from build123d import *

# Parameters (mm, degrees)
SKETCH_1_R      = 2.5
EXTRUDE_1_DEPTH = 4


with BuildPart() as part:
    # 草图1 → 凸台-拉伸1 (new body)
    with BuildSketch(Plane.XY):
        with BuildLine():
            Line((-3.705318961, 51.777526587), (-4.499753228, 50.342391759))
            ThreePointArc((-4.499753228, 50.342391759), (-4.72372629, 49.780297575), (-4.8, 49.180050853))
            Line((-4.8, 49.180050853), (-4.8, 14.202498322))
            ThreePointArc((-4.8, 14.202498322), (-4.74482021, 13.6908166), (-4.581818179, 13.20266362))
            Line((-4.581818179, 13.20266362), (-4.112355754, 12.178212626))
            ThreePointArc((-4.112355754, 12.178212626), (-3.746152658, 10.910853721), (-3.111838791, 9.754156171))
            ThreePointArc((-3.111838791, 9.754156171), (-2.4, 7.5), (-3.111838791, 5.245843829))
            ThreePointArc((-3.111838791, 5.245843829), (-3.921495991, 3.606788208), (-4.2, 1.8))
            Line((-4.2, 1.8), (-4.2, 0))
            ThreePointArc((-4.2, 0), (0, -4.2), (4.2, 0))
            Line((4.2, 0), (4.2, 1.8))
            ThreePointArc((4.2, 1.8), (3.921495991, 3.606788208), (3.111838791, 5.245843829))
            ThreePointArc((3.111838791, 5.245843829), (2.4, 7.5), (3.111838791, 9.754156171))
            ThreePointArc((3.111838791, 9.754156171), (3.921495991, 11.393211792), (4.2, 13.2))
            Line((4.2, 13.2), (4.2, 49.8))
            ThreePointArc((4.2, 49.8), (1.019230191, 53.874453315), (-3.705318961, 51.777526587))
        make_face()
        Circle(SKETCH_1_R, mode=Mode.SUBTRACT)
        with BuildLine():
            Line((-3, 45.643078062), (-3, 15))
            ThreePointArc((-3, 15), (2.449489743, 13.267949192), (-1, 17.828427125))
            ThreePointArc((-1, 17.828427125), (-1.546410162, 17.904214601), (-1.8, 18.39411255))
            Line((-1.8, 18.39411255), (-1.8, 45.643078062))
            ThreePointArc((-1.8, 45.643078062), (-2.4, 46.243078062), (-3, 45.643078062))
        make_face(mode=Mode.SUBTRACT)
        with BuildLine():
            Line((1.5, 48.477124344), (1.5, 51.122875656))
            ThreePointArc((1.5, 51.122875656), (-2, 49.8), (1.5, 48.477124344))
        make_face(mode=Mode.SUBTRACT)
    extrude(amount=EXTRUDE_1_DEPTH)


solid = part.part
Geometry check sheet. Reference: the model listing, model coordinates, mm. A direction names the side the tool comes from. Give positions to 0.01 mm unless a question says otherwise; leave off trailing zeros. Order: outer loops, then holes, each group sorted by start corner. A loop starts at its lowest first (then second) coordinate and runs counter-clockwise, first axis right, second up.
1) Cross-section at B-B (y = 37). Record the boundary of the cut face in (x, z).
Results are:
outline: (-4.8, 0) - (-3, 0) - (-3, 4) - (-4.8, 4) - close; (-1.8, 0) - (4.2, 0) - (4.2, 4) - (-1.8, 4) - close
2) Gauge pin test, flat ends, axial feed: pin 1 (4.5 mm diameter, centred on x = 0, y = 49.8, fed in from +Z); pin 2 (0.9 mm diameter, centred on y = 0.5, z = 2.5, fed in from -X); pin 3 (1.5 mm diameter, centred on y = 12.5, z = 1.5, fed in from -X); pin 4 (2 mm diameter, centred on x = -3.5, z = 2, fed in from +Y). Record the tip position at first contact, or that the pin passes through.
Results are:
pin 1: stops at z = 4
pin 2: stops at x = -4.2
pin 3: stops at x = -4.6
pin 4: stops at y = 53.17
3) Tool access check on faces 4 (the cylindrical face through (-3.914, 3.631, 1.972)), 5 (the cylindrical face through (-2.387, 46.243, 1.972)), 6 (the cylindrical face through (3.93, 3.58, 1.97)), 7 (the flat face through (-4.2, 1, 2)). Record the directions out of +Z, -Z, +X, -X, +Y, -Y that give a thin tool (end or side, any length) a straight path to the whole face; none if there is none.
Results are:
face 4: +Z, -Z, -X
face 5: +Z, -Z
face 6: +Z, -Z, +X
face 7: +Z, -Z, -X, -Y
4) Draft check along Y on faces 1 (the cylindrical face through (-4.72, 49.79, 1.97)), 2 (the flat face through (-3, 31, 2)), 3 (the cylindrical face through (-4.746, 13.698, 1.972)). Enter one of: released by +Y, released by -Y, zero draft, split by the parting line, or undercut.
Results are:
face 1: released by +Y
face 2: undercut
face 3: released by -Y
5) Material ranges on probe 1 along Y at (x, z) = (0, 2.55); probe 2 along X at (y, z) = (19, 2.85); probe 3 along Y at (x, z) = (-0.5, 1.8), recorded low to high.
Results are:
probe 1: y = -4.2 to -2.5, 2.5 to 12, 18 to 47.8, 51.8 to 54
probe 2: x = -4.8 to -3, -1.8 to 4.2
probe 3: y = -4.17 to -2.45, 2.45 to 12.04, 17.96 to 47.86, 51.74 to 53.97
6) Cross-section at A-A (x = 0). Record the boundary of the cut face in (y, z), then the cut area to 3 significant figures.
Results are:
outline: (-4.2, 0) - (-2.5, 0) - (-2.5, 4) - (-4.2, 4) - close; (2.5, 0) - (12, 0) - (12, 4) - (2.5, 4) - close; (18, 0) - (47.8, 0) - (47.8, 4) - (18, 4) - close; (51.8, 0) - (54, 0) - (54, 4) - (51.8, 4) - close
area: 173 mm2
7) Cross-section at C-C (z = 1.85). Give the number of separate pieces and of enclosed holes in the cut face, then the cut area to 3 significant figures.
Results are:
separate pieces: 1
enclosed holes: 3
area: 382 mm2
